from build123d import *

# Parameters (mm, degrees)
F1_DEPTH = 25.4
F2_R     = 6.35
F3_R     = 1.5875
F4_DEPTH = 12.7


with BuildPart() as f1:
    # F0 (on Top) → F1 (new body)
    with BuildSketch(Plane.XY):
        with BuildLine():
            ThreePointArc((127, 38.1), (100.961793, 100.961793), (38.1, 127))
            Line((38.1, 127), (-38.1, 127))
            ThreePointArc((-38.1, 127), (-100.961793, 100.961793), (-127, 38.1))
            Line((-127, 38.1), (-127, -38.1))
            ThreePointArc((-127, -38.1), (-100.961793, -100.961793), (-38.1, -127))
            Line((-38.1, -127), (38.1, -127))
            ThreePointArc((38.1, -127), (100.961793, -100.961793), (127, -38.1))
            Line((127, -38.1), (127, 38.1))
        make_face()
    extrude(amount=F1_DEPTH)

    # F2
    f2_edges = [f1.edges().sort_by_distance(p)[0] for p in [
        (-100.961793, -100.961793, 25.4),
        (-100.961793, -100.961793, 0),
    ]]
    fillet(f2_edges, radius=F2_R)

    # F3 (on face) → F4 (cut)
    with BuildSketch(Plane(origin=(0, 0, 0), x_dir=(1, 0, 0), z_dir=(0, 0, -1))):
        with Locations((-114.3, 36.240128)):
            Circle(F3_R)
        with Locations((114.3, 36.240128)):
            Circle(F3_R)
        with Locations((114.3, -38.1)):
            Circle(F3_R)
        with Locations((-114.3, -38.1)):
            Circle(F3_R)
    extrude(amount=-F4_DEPTH, mode=Mode.SUBTRACT)


solid = f1.part
Build history of the part. All positions in model axes, mm. Round coordinates to 2 decimals unless told otherwise and drop trailing zeros. Use CSV: the item, a comma, the result in double quotes.
1. Wall check: probe 1 along X at (y, z) = (38.1, 8.5); probe 2 along Y at (x, z) = (114.3, 3.5); probe 3 along X at (y, z) = (71, 18.75). Give the ranges that are in metal, low to high. Write a range as from..to.
Reply:
probe 1,"x = -127..-115.89, -112.71..112.71, 115.89..127"
probe 2,"y = -82.56..-37.83, -34.65..36.51, 39.69..82.56"
probe 3,"x = -120.69..120.69"
2. Flat gauge pins, fed straight in: pin 1 (1.6 mm diameter, centred on x = -114.5, y = 37.5, fed in from -Z); pin 2 (2 mm diameter, centred on x = 81.5, z = 7.5, fed in from -Y); pin 3 (1.5 mm diameter, centred on x = 65.5, z = 3, fed in from -Y). Where does each tip first touch, or does it go through?
Reply:
pin 1,"stops at z = 12.7"
pin 2,"stops at y = -116.24"
pin 3,"stops at y = -122.16"
3. Two-plate mould, pull along Z, no slides. Class faces 1 (the face through (-0.53, 125.19, 1.91)), 2 (the face through (0.53, -125.19, 23.49)), 3 (the face through (-127, 1, 13)): +Z half, -Z half, draft (parallel to the pull), parting line (faces both ways), or undercut.
Reply:
face 1,"-Z half"
face 2,"+Z half"
face 3,"draft"
